from build123d import *

# Parameters (mm, degrees)
SKETCH1_W           = 7
SKETCH1_H           = 7
BOSS_EXTRUDE1_DEPTH = 100
SKETCH3_W           = 80
SKETCH3_H           = 80
BOSS_EXTRUDE2_DEPTH = 5
BOSS_EXTRUDE5_DEPTH = 7
SKETCH11_W          = 20
SKETCH11_H          = 25
BOSS_EXTRUDE6_DEPTH = 10


with BuildPart() as part:
    # Sketch1 → Boss-Extrude1 (new body)
    with BuildSketch(Plane.XY):
        Rectangle(SKETCH1_W, SKETCH1_H)
    extrude(amount=BOSS_EXTRUDE1_DEPTH)

    # Sketch3 → Boss-Extrude2 (add)
    with BuildSketch(Plane(origin=(0, 3.5, 0), x_dir=(1, 0, 0), z_dir=(0, 1, 0))):
        with Locations((-43.5, -60)):
            Rectangle(SKETCH3_W, SKETCH3_H)
    extrude(amount=-BOSS_EXTRUDE2_DEPTH)

    # Sketch8 → Boss-Extrude5 (add)
    with BuildSketch(Plane.XZ.offset(3.5)):
        Polygon((-3.5, 20), (-6.5, 20), (-18.5, 4), (-3.5, 4), align=None)
    extrude(amount=-BOSS_EXTRUDE5_DEPTH)

    # Sketch11 → Boss-Extrude6 (add)
    with BuildSketch(Plane(origin=(3.5, 0, 0), x_dir=(0, 0, -1), z_dir=(1, 0, 0))):
        with Locations((-14.137320527, 0)):
            Rectangle(SKETCH11_W, SKETCH11_H)
    extrude(amount=BOSS_EXTRUDE6_DEPTH)


solid = part.part
Geometry: final body of the model. Coordinates: model frame, mm. A direction names the side the tool comes from. Round coordinates to 2 decimals unless told otherwise and drop trailing zeros. Loops run counter-clockwise (first coordinate to the right, second up) from the corner with the lowest first, then second, coordinate; pieces in that order, holes last.
Q1. Section D-D on y = -9. Return loops of the section in (x, z), plus the area to 3 significant figures.
Q2. Section C-C on x = -33. Return loops of the section in (y, z), plus the area to 3 significant figures.
Q3. Pull-direction query (Z, two-part tool) for faces 1 (the flat face through (-12.416, -0.049, 12.112)), 2 (the flat face through (8, 0, 24.137)), 3 (the flat face through (-83.5, 1, 61)); classes: released by +Z, released by -Z, zero draft, split by the parting line, or undercut.
Q4. Access query for faces 4 (the flat face through (3.5, -8, 14)), 5 (the flat face through (-3.5, 0, 2)), 6 (the flat face through (3.5, 0, 62)), 7 (the flat face through (-44, -1.5, 59)), 8 (the flat face through (8, 0, 4.137)). Directions: +Z, -Z, +X, -X, +Y, -Y. A direction counts if a zero-diameter tool reaches every point of the face in a straight line with its end or side. Return the directions, or none.
Q5. Material intervals for L1, parallel to Y at x = -41.5, z = 85; L2, parallel to X at y = 6.5, z = 21.5; L3, parallel to Y at x = -1.5, z = 87.5, sorted ascending.
Q6. Section A-A on x = -8. Return loops of the section in (y, z).
Q7. Pin query (flat end, axial travel): P1, Ø5, axis at x = 8.5, y = -1, coming from the +Z side; P2, Ø7, axis at y = 6.5, z = 16, coming from the -X side; P3, Ø4, axis at x = -11, y = -4.5, coming from the -Z side; P4, Ø24, axis at x = -4.5, z = 32.5, coming from the -Y side. Return the tip coordinate at first contact, or that it passes through.
Q8. Section B-B on z = 14. Return loops of the section in (x, y), plus the area to 4 significant figures.
Evaluation:
1. outline: (3.5, 4.14) - (13.5, 4.14) - (13.5, 24.14) - (3.5, 24.14) - close
1. area: 200 mm2
2. outline: (-1.5, 20) - (3.5, 20) - (3.5, 100) - (-1.5, 100) - close
2. area: 400 mm2
3. face 1: undercut
3. face 2: released by +Z
3. face 3: zero draft
4. face 4: +Z, -Z, -X, -Y
4. face 5: -Z, -X, +Y, -Y
4. face 6: +Z, +X, +Y, -Y
4. face 7: +Z, -X, -Y
4. face 8: -Z, +X, +Y, -Y
5. L1: y = -1.5 to 3.5
5. L2: x = 3.5 to 13.5
5. L3: y = -3.5 to 3.5
6. outline: (-3.5, 4) - (3.5, 4) - (3.5, 18) - (-3.5, 18) - close; (-1.5, 20) - (3.5, 20) - (3.5, 100) - (-1.5, 100) - close
7. P1: stops at z = 24.14
7. P2: stops at x = -10.85
7. P3: stops at z = 4
7. P4: stops at y = -12.5
8. outline: (-11, -3.5) - (3.5, -3.5) - (3.5, -12.5) - (13.5, -12.5) - (13.5, 12.5) - (3.5, 12.5) - (3.5, 3.5) - (-11, 3.5) - close
8. area: 351.5 mm2
